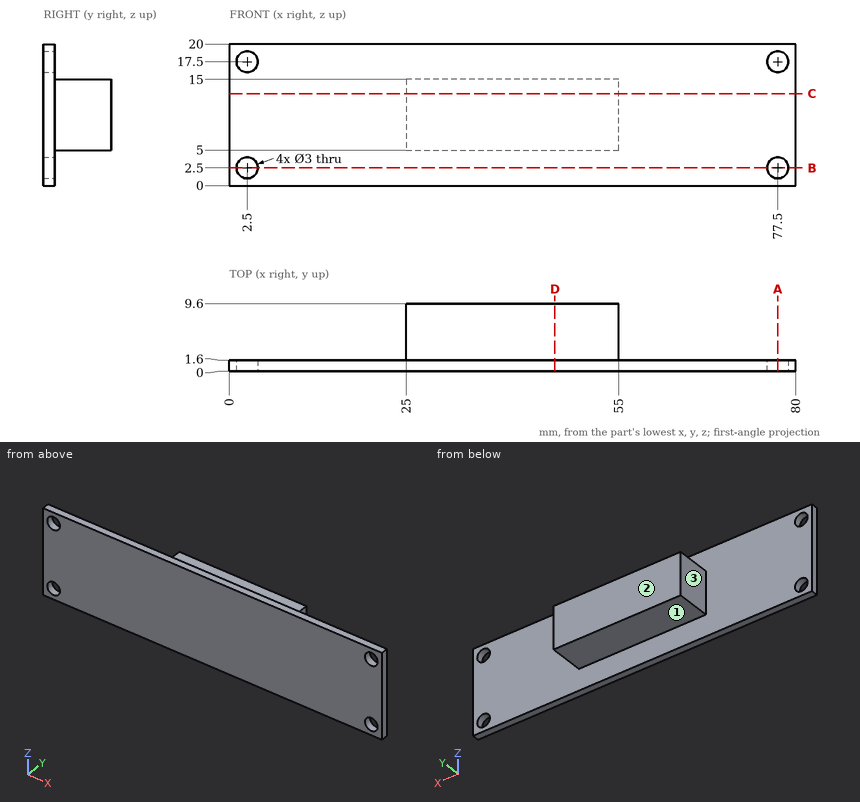
Here's the drawing with two shaded views (mm, measured from the low corner). I have some questions. A direction names the side the tool comes from. Give positions to 0.01 mm unless a question says otherwise; leave off trailing zeros. Order: outer loops, then holes, each group sorted by start corner. A loop starts at its lowest first (then second) coordinate and runs counter-clockwise, first axis right, second up. Notation, with made-up numbers: M 48.5,31.25 L 106.5,31.25 A17 cw 106.5,60.25 Z; hole C -6,20 d2. An arc over 180 degrees is marked long. One line per item, written item: value.
1) I want a section at D-D, the plane x = 46. List the corners of the cut face in (y, z) for me.
Answer sheet:
outline: M 0,0 L 1.6,0 L 1.6,5 L 9.6,5 L 9.6,15 L 1.6,15 L 1.6,20 L 0,20 Z
2) On a 3-axis mill with a long thin cutter (end or side, diameter ignored), from which of +Z, -Z, +X, -X, +Y, -Y can I reach the whole of each face in a straight line? I mean the marked faces 1, 2 and 3. Say none if no direction works.
Answer sheet:
face 1: -Z, +X, -X, +Y
face 2: +Z, -Z, +X, -X, +Y
face 3: +Z, -Z, -X, +Y
3) I want a section at B-B, the plane z = 2.5. List the corners of the cut face in (x, y) for me.
Answer sheet:
outline: M 0,0 L 1,0 L 1,1.6 L 0,1.6 Z; M 4,0 L 76,0 L 76,1.6 L 4,1.6 Z; M 79,0 L 80,0 L 80,1.6 L 79,1.6 Z
4) For P1, Ø2, axis at y = 3, z = 13, coming from the -X side; P2, Ø4, axis at y = 5.5, z = 8.5, coming from the +X side; P3, Ø1.5, axis at y = 8, z = 4, coming from the +X side; P4, Ø3.5, axis at x = 2.5, z = 2.5, coming from the +Y side, each with a flat end and sliding along its axis, tell me the tip position at first contact or that it passes through.
Answer sheet:
P1: stops at x = 25
P2: stops at x = 55
P3: passes through
P4: stops at y = 1.6
5) I want a section at C-C, the plane z = 13. List the corners of the cut face in (x, y) for me.
Answer sheet:
outline: M 0,0 L 80,0 L 80,1.6 L 55,1.6 L 55,9.6 L 25,9.6 L 25,1.6 L 0,1.6 Z
6) Please list where these lines run through material, in increasing order: line 1 along Z through (x, y) = (77.5, 0.5); line 2 along X through (y, z) = (1.2, 17.5); line 3 along Y through (x, z) = (16, 11).
Answer sheet:
line 1: z = 0 to 1, 4 to 16, 19 to 20
line 2: x = 0 to 1, 4 to 76, 79 to 80
line 3: y = 0 to 1.6
7) I want a section at A-A, the plane x = 77.5. List the corners of the cut face in (y, z) for me, plus the area to 3 significant figures.
Answer sheet:
outline: M 0,0 L 1.6,0 L 1.6,1 L 0,1 Z; M 0,4 L 1.6,4 L 1.6,16 L 0,16 Z; M 0,19 L 1.6,19 L 1.6,20 L 0,20 Z
area: 22.4 mm^2
